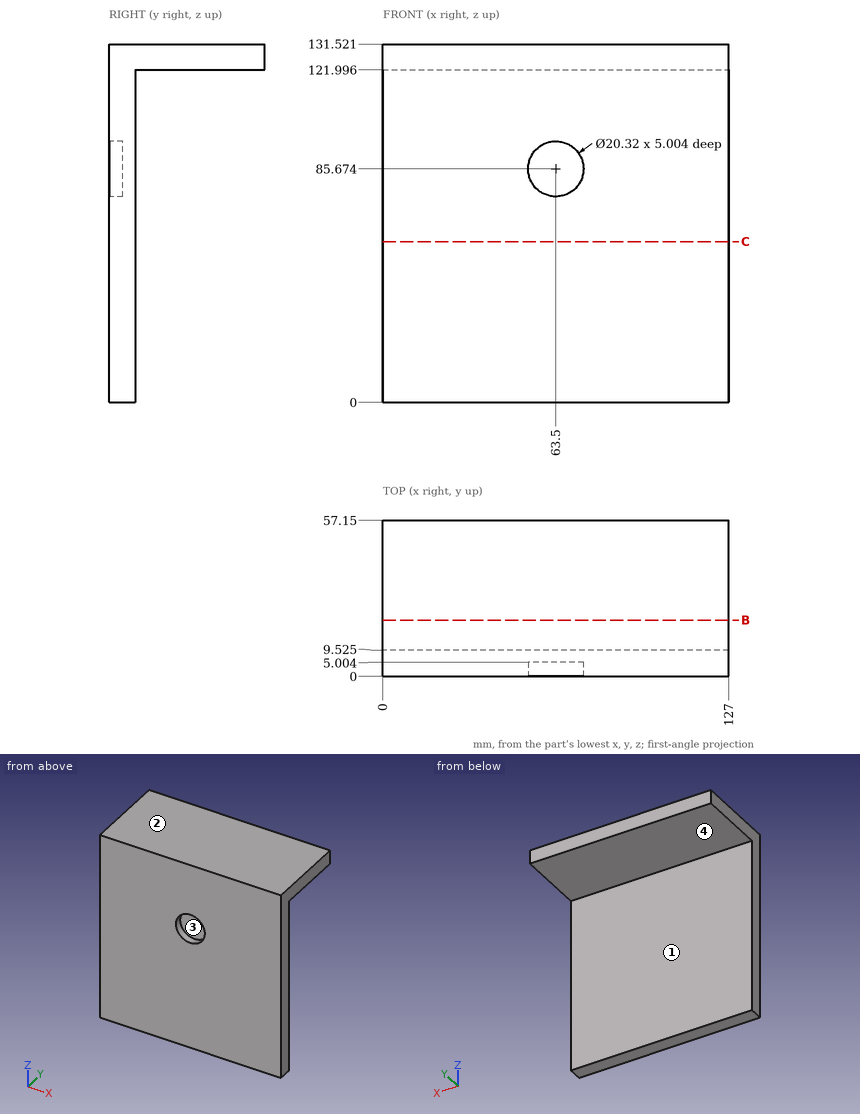
Design review of the part shown in the three views and the two pictorial views. Dimensions are in mm from the part's minimum x, y and z. A direction names the side the tool comes from. Give positions to 0.01 mm unless a question says otherwise; leave off trailing zeros. Loops run counter-clockwise (first coordinate to the right, second up) from the corner with the lowest first, then second, coordinate; pieces in that order, holes last. Notation, with made-up numbers: (72, 53) - (130, 53) arc R5 cw to (130, 57) - close; hole circle Ø1 at (8, 24.25). An arc over 180 degrees is marked (long way). Answer as a JSON object with one key per item and string values.
Q1. Mouldability with a two-part tool opening along X and no side actions: class the marked faces 3 and 4 as +X half, -X half, draft (parallel to the pull), parting line (faces both ways), or undercut.
Worked out:
{"face 3": "undercut", "face 4": "draft"}
Q2. Add section C-C on z = 59. State the section outline as (x, y) points (3 decimals).
Worked out:
{"outline": "(0, 0) - (127, 0) - (127, 9.525) - (0, 9.525) - close"}
Q3. To check wall thickness, follow line 1 along Z through (x, y) = (63.5, 3.4); line 2 along Z through (x, y) = (110, 37); line 3 along Y through (x, z) = (109, 34.5) (3 decimals). State the ranges of each line that lie inside material, in increasing order.
Worked out:
{"line 1": "z = 0 to 75.51, 95.83 to 131.52", "line 2": "z = 122 to 131.52", "line 3": "y = 0 to 9.525"}
Q4. Add section B-B on y = 20.5. State the section outline as (x, z) points.
Worked out:
{"outline": "(0, 122) - (127, 122) - (127, 131.52) - (0, 131.52) - close"}
Q5. Insertion check: pin 1 (6 mm diameter, centred on x = 61, z = 90.5, fed in from -Y); pin 2 (10 mm diameter, centred on x = 99.5, z = 95, fed in from +Y) (3 decimals); pin 3 (14.5 mm diameter, centred on x = 46.5, y = 35.5, fed in from -Z). Each pin has a flat end and moves straight along its axis. Give the tip position at first contact, or say it passes through.
Worked out:
{"pin 1": "stops at y = 5", "pin 2": "stops at y = 9.525", "pin 3": "stops at z = 122"}
Q6. For the marked faces 1 and 2, list the 3-axis set-ups (+Z, -Z, +X, -X, +Y, -Y) from which the entire face can be reached by the end or side of a thin tool; tool diameter is ignored.
Worked out:
{"face 1": "-Z, +X, -X, +Y", "face 2": "+Z, +X, -X, +Y, -Y"}
